Geometry check sheet. Reference: the model listing, model coordinates, mm. A direction names the side the tool comes from. Give positions to 0.01 mm unless a question says otherwise; leave off trailing zeros. Order: outer loops, then holes, each group sorted by start corner. A loop starts at its lowest first (then second) coordinate and runs counter-clockwise, first axis right, second up.
from build123d import *

# Parameters (mm, degrees)
F1_DEPTH = 5
F2_SIZE  = 7
F3_W     = 7
F3_H     = 3
F4_DEPTH = 15
F5_SIZE  = 3


with BuildPart() as f1:
    # F0 (on Front) → F1 (new body)
    with BuildSketch(Plane.XZ):
        with BuildLine():
            ThreePointArc((3, 2.645751), (3.741657, 1.414214), (4, 0))
            ThreePointArc((4, 0), (-1.414214, -3.741657), (-3, 2.645751))
            Line((-3, 2.645751), (-3, 8))
            Line((-3, 8), (-10, 8))
            Line((-10, 8), (-10, -7))
            Line((-10, -7), (0, -7))
            Line((0, -7), (10, -7))
            Line((10, -7), (10, 8))
            Line((10, 8), (3, 8))
            Line((3, 8), (3, 2.645751))
        make_face()
    extrude(amount=F1_DEPTH)

    # F2
    f2_edges = [f1.edges().sort_by_distance(p)[0] for p in [
        (-10, -2.5, -7),
        (10, -2.5, -7),
    ]]
    chamfer(f2_edges, length=F2_SIZE)

    # F3 (on face) → F4 (join)
    with BuildSketch(Plane(origin=(0, 0, 0), x_dir=(-1, 0, 0), z_dir=(0, 1, 0))):
        with Locations((-6.5, 6.5)):
            Rectangle(F3_W, F3_H)
        with Locations((6.5, 6.5)):
            Rectangle(F3_W, F3_H)
    extrude(amount=F4_DEPTH)

    # F5
    f5_edges = [f1.edges().sort_by_distance(p)[0] for p in [
        (-3, 5, 8),
        (3, 5, 8),
    ]]
    chamfer(f5_edges, length=F5_SIZE)


solid = f1.part
Item 1: Gauge pin test, flat ends, axial feed: pin 1 (3.5 mm diameter, centred on x = -7.5, y = 6, fed in from -Z); pin 2 (3 mm diameter, centred on x = 6.5, z = 3, fed in from +Y). Record the tip position at first contact, or that the pin passes through.
Reported:
pin 1: stops at z = 5
pin 2: stops at y = 0
Item 2: Scan lines: L1, parallel to X at y = 1, z = 7; L2, parallel to Y at x = 5, z = -2.25; L3, parallel to Z at x = 0, y = -2.35. Record each from-to range of solid material in increasing order.
Reported:
L1: x = -10 to -5, 5 to 10
L2: y = -5 to 0
L3: z = -7 to -4
Item 3: Sectioned sample at D-D (x = 4.5). Enter the section's corners in (y, z), and give its area (3 significant figures).
Reported:
outline: (-5, -5.5) - (0, -5.5) - (0, 5) - (15, 5) - (15, 6.5) - (-5, 6.5) - close
area: 82.5 mm2
Item 4: Set-up check for faces 1 (the flat face through (-3, -2, 4)), 2 (the flat face through (7, -2, -3)), 3 (the flat face through (7, 7, 5)): record each of +Z, -Z, +X, -X, +Y, -Y from which the full face is reachable in a straight line by a thin tool's end or side.
Reported:
face 1: +Z, +Y, -Y
face 2: -Z, +X, +Y, -Y
face 3: -Z, +X, -X, +Y
Item 5: Sectioned sample at C-C (y = -1.5). Enter the section's corners in (x, z), and give its area (3 significant figures).
Reported:
outline: (-10, 0) - (-3, -7) - (3, -7) - (10, 0) - (10, 8) - (6, 8) - (3, 5) - (3, 2.65) arc R4 cw to (4, 0) arc R4 cw (long way) to (-3, 2.65) - (-3, 5) - (-6, 8) - (-10, 8) - close
area: 165 mm2
Item 6: Sectioned sample at A-A (y = 5.75). Enter the section's corners in (x, z), and give its area (3 significant figures).
Reported:
outline: (-10, 5) - (-3, 5) - (-6, 8) - (-10, 8) - close; (3, 5) - (10, 5) - (10, 8) - (6, 8) - close
area: 33.0 mm2
Item 7: Sectioned sample at B-B (z = 5.5). Enter the section's corners in (x, y).
Reported:
outline: (-10, -5) - (-3.5, -5) - (-3.5, 15) - (-10, 15) - close; (3.5, -5) - (10, -5) - (10, 15) - (3.5, 15) - close
